For this review, take the finished solid that the model builds, in its own axes (mm). Face numbers are marked on the shaded views. A direction names the side the tool comes from. Coordinates: 2 decimals unless noted, no trailing zeros. Write each loop counter-clockwise with the first axis right and the second up, starting at its lowest first coordinate (ties: lowest second). Pieces come first, ordered by that corner, then holes. Notation, with made-up numbers: (40, 85.25) -> (70, 85.25) arc R31 cw to (70, 115.25) -> close; hole circle Ø6 at (31, -8.75). An arc over 180 degrees is marked (long way). Put each result on its own line as item: value. Start each with the question number.
Item 1: Consider section A-A on x = -6.5. Give the boundary of the cut face in (y, z) (1 decimal).
Item 2: Consider section C-C on z = -13. Give the boundary of the cut face in (x, y).
Item 3: Insertion check: P1, Ø2.5, axis at y = 6.5, z = -56, coming from the +X side; P2, Ø6, axis at x = -29.5, z = -25, coming from the +Y side; P3, Ø0.6, axis at x = -1.5, y = 7.5, coming from the +Z side; P4, Ø3, axis at x = -17, z = -38.5, coming from the -Y side. Each pin has a flat end and moves straight along its axis. Give the tip position at first contact, or say it passes through.
Item 4: To check wall thickness, follow L1, parallel to Z at x = -6.5, y = 14.85; L2, parallel to Z at x = -32.5, y = 0.95; L3, parallel to Y at x = -5.5, z = -32.5. State the ranges of each line that lie inside material, in increasing order.
Item 5: For the marked faces 1, 2, 3 and 4, list the 3-axis set-ups (+Z, -Z, +X, -X, +Y, -Y) from which the entire face can be reached by the end or side of a thin tool; tool diameter is ignored.
Item 6: Consider section B-B on z = -5. Give the boundary of the cut face in (x, y).
Item 7: Consider section D-D on x = -25. Give the boundary of the cut face in (y, z).
Autodesk Inventor part; units mm, degrees
ref_plane "YZ Plane" through (0, 0, 0) normal (1, 0, 0) x (0, 1, 0)
ref_plane "XZ Plane" through (0, 0, 0) normal (0, 1, 0) x (-1, 0, 0)
ref_plane "XY Plane" through (0, 0, 0) normal (0, 0, 1) x (1, 0, 0)
sketch "Sketch1" plane through (0, 0, 0) normal (0, 1, 0) x (-1, 0, 0)
  line L0 (0, 0) -> (40, 0)
  line L1 (40, 0) -> (40, -65)
  line L2 (40, -65) -> (0, -65)
  line L3 (0, -65) -> (0, 0)
  dimension "d0" = 40
  dimension "d1" = 65
extrude "Extrusion1" add sketch "Sketch1" along normal blind 16
sketch "Sketch2" plane through (-40, 0, 0) normal (0, 0, 1) x (1, 0, 0)
  line L0 (0, 16) -> (40, 16)
  line L1 (0, 16) -> (20, 16)
  line L2 (20, 16) -> (20, 3.5)
  line L3 (20, 3.5) -> (0, 3.5)
  line L4 (0, 3.5) -> (0, 16)
  line L5 (40, 0) -> (0, 0)
  dimension "d4" = 20
  dimension "d5" = 3.5
extrude "Extrusion2" cut sketch "Sketch2" against normal through all
sketch "Sketch3" plane through (0, 0, 0) normal (0, -1, 0) x (1, 0, 0)
  line L0 (-32.5, -58) -> (-32.5, -13) construction
  line L1 (-6.5, -55) -> (-6.5, -5) construction
  line L2 (-40, -65) -> (0, -65) construction
  line L3 (0, 0) -> (-40, 0) construction
  line L4 (0, -65) -> (0, 0) construction
  line L5 (-40, 0) -> (-40, -65) construction
  dimension "d8" = 45
  dimension "d9" = 50
  dimension "d10" = 7
  dimension "d11" = 5
  dimension "d12" = 6.5
  dimension "d13" = 7.5
hole "Hole1" at (-32.5, 0, -58) at (-32.5, 0, -13) at (-6.5, 0, -55) at (-6.5, 0, -5) direction (0, 1, 0) diameter 3.4 end through all
sketch "Sketch4" plane through (0, 0, 0) normal (1, 0, 0) x (0, 0, -1)
  line L0 (38.5, 6.5) -> (38.5, 9.5) construction
  line L1 (39.35, 6.5) -> (39.35, 9.5)
  line L2 (37.65, 9.5) -> (37.65, 6.5)
  arc A0 (37.65, 6.5) -> (39.35, 6.5) centre (38.5, 6.5) ccw
  arc A1 (39.35, 9.5) -> (37.65, 9.5) centre (38.5, 9.5) ccw
  line L3 (26.5, 6.5) -> (26.5, 9.5) construction
  line L4 (27.35, 6.5) -> (27.35, 9.5)
  line L5 (25.65, 9.5) -> (25.65, 6.5)
  arc A2 (25.65, 6.5) -> (27.35, 6.5) centre (26.5, 6.5) ccw
  arc A3 (27.35, 9.5) -> (25.65, 9.5) centre (26.5, 9.5) ccw
  line L6 (0, 0) -> (0, 16) construction
  line L7 (65, 0) -> (65, 16) construction
  line L8 (38.5, 8) -> (26.5, 8) construction
  line L9 (65, 0) -> (0, 0) construction
  line L10 (0, 16) -> (65, 16) construction
  line L11 (65, 0) -> (40.5, 0)
  line L12 (40.5, 0) -> (40.5, 13)
  line L13 (40.5, 13) -> (65, 13)
  line L14 (65, 13) -> (65, 0)
  line L15 (24.5, 0) -> (0, 0)
  line L16 (0, 0) -> (0, 13)
  line L17 (0, 13) -> (24.5, 13)
  line L18 (24.5, 13) -> (24.5, 0)
  point P0 (32.5, 8)
  dimension "d21" = 12
  dimension "d22" = 6
  dimension "d23" = 65
  dimension "d24" = 32.5
  dimension "d25" = 3
  dimension "d26" = 3
  dimension "d27" = 0.85
  dimension "d28" = 0.85
  dimension "d29" = 0
  dimension "d30" = 16
  dimension "d31" = 8
  dimension "d32" = 3
  dimension "d33" = 3
  dimension "d34" = 16
  dimension "d35" = 8
extrude "Extrusion3" cut sketch "Sketch4" against normal blind 2 contours A0 L2 A1 L1 | A2 L5 A3 L4
extrude "Extrusion4" cut sketch "Sketch4" against normal blind 17 contours L11 L12 L13 L14 | L15 L16 L17 L18
fillet "Fillet1" radius 2 14 edges at (-8.5, 0, -40.5) (-8.5, 0, -24.5) (-40, 1.75, -65) (-40, 1.75, 0) (0, 14.5, 0) (0, 14.5, -65) (-17, 0, -52.75) (-17, 0, -12.25) (-17, 6.5, -40.5) (-17, 6.5, -24.5) (-17, 13, -52.75) (-8.5, 13, -40.5) (-17, 13, -12.25) (-8.5, 13, -24.5)
hole "Hole2" at (0, 8, -32.5) direction (-1, 0, 0) diameter 6.125 depth 10 tip angle 118
equation "\"d26\" = d25"
equation "\"d28\" = d27"
properties part number "Dual Camera Mount"
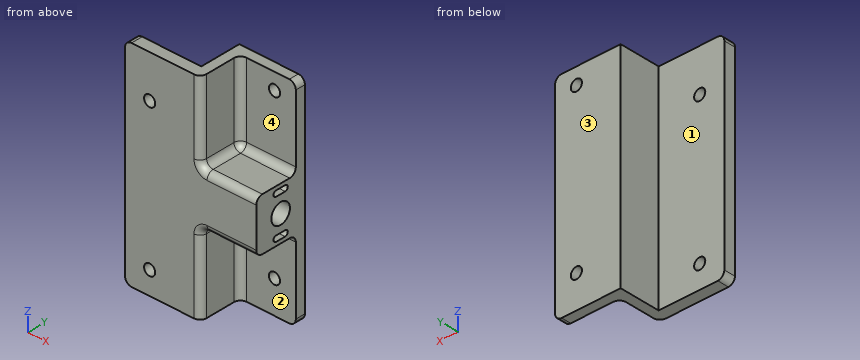
Return value:
1. outline: (0, -38.5) arc R2 ccw to (2, -40.5) -> (11, -40.5) arc R2 cw to (13, -42.5) -> (13, -53.3) -> (16, -53.3) -> (16, -6.7) -> (13, -6.7) -> (13, -22.5) arc R2 cw to (11, -24.5) -> (2, -24.5) arc R2 ccw to (0, -26.5) -> close; (13, -65) -> (16, -65) -> (16, -56.7) -> (13, -56.7) -> close; (13, -3.3) -> (16, -3.3) -> (16, 0) -> (13, 0) -> close; hole circle Ø6.1 at (8, -32.5)
2. outline: (-40, 0) -> (-34.2, 0) -> (-34.2, 3.5) -> (-40, 3.5) -> close; (-30.8, 0) -> (-19, 0) arc R2 ccw to (-17, 2) -> (-17, 11) arc R2 cw to (-15, 13) -> (0, 13) -> (0, 16) -> (-20, 16) -> (-20, 3.5) -> (-30.8, 3.5) -> close
3. P1: x = -17
3. P2: y = 3.5
3. P3: z = -24.5
3. P4: y = 0
4. L1: -65 to -56.7, -53.3 to -6.7, -3.3 to 0
4. L2: -65 to -59.7, -56.3 to -14.7, -11.3 to 0
4. L3: 0 to 4.94, 11.06 to 16
5. face 1: +Z, -Z, -X, +Y
5. face 2: -Z, +X, -Y
5. face 3: +Z, -Z, +X, -X, +Y
5. face 4: +Z, +X, -Y
6. outline: (-40, 0) -> (-19, 0) arc R2 ccw to (-17, 2) -> (-17, 11) arc R2 cw to (-15, 13) -> (-8.2, 13) -> (-8.2, 16) -> (-20, 16) -> (-20, 3.5) -> (-40, 3.5) -> close; (-4.8, 13) -> (0, 13) -> (0, 16) -> (-4.8, 16) -> close
7. outline: (0, -65) -> (3.5, -65) -> (3.5, 0) -> (0, 0) -> close
